Here's the drawing with two shaded views (mm, measured from the low corner). I have some questions. Give positions to 0.01 mm unless a question says otherwise; leave off trailing zeros. Loops run counter-clockwise (first coordinate to the right, second up) from the corner with the lowest first, then second, coordinate; pieces in that order, holes last.
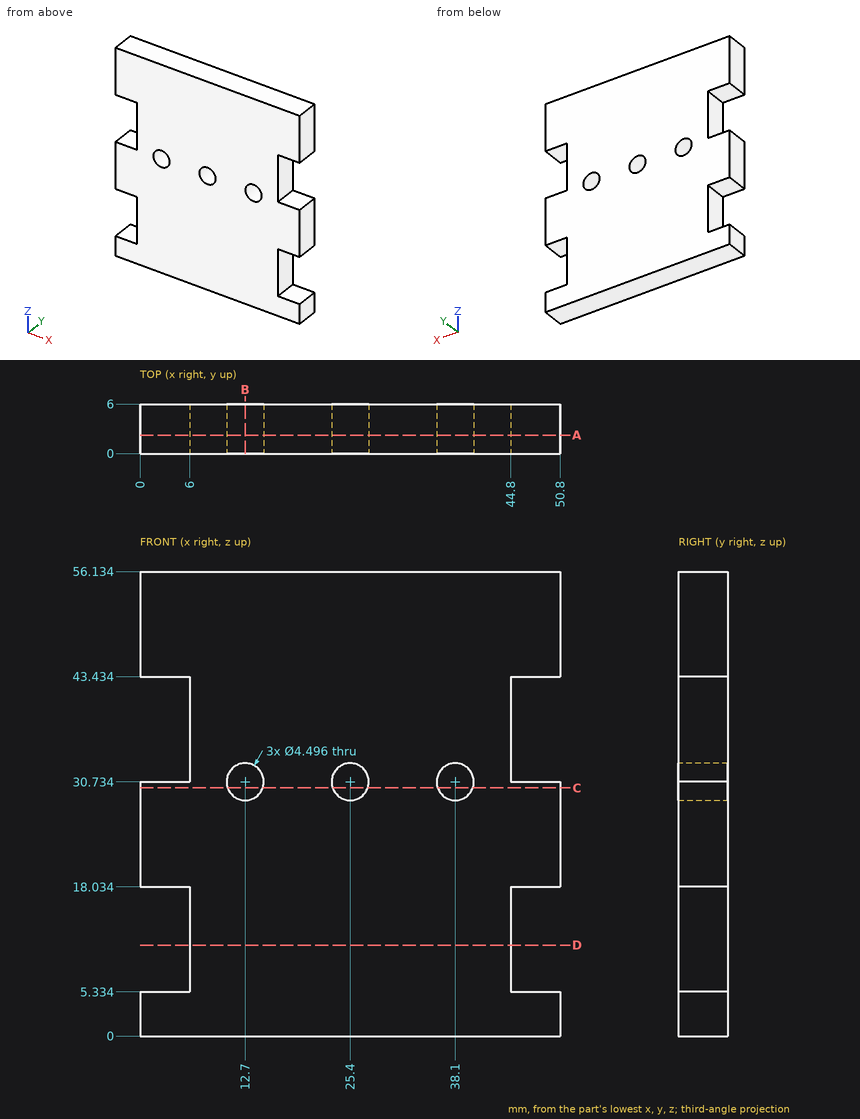
(1) Please list where these lines run through material, in increasing order: probe 1 along X at (y, z) = (2.5, 29); probe 2 along Z at (x, y) = (38.1, 2.35); probe 3 along X at (y, z) = (2, 12).
Returned:
probe 1: x = 0 to 11.27, 14.13 to 23.97, 26.83 to 36.67, 39.53 to 50.8
probe 2: z = 0 to 28.49, 32.98 to 56.13
probe 3: x = 6 to 44.8
(2) Will these pins go through, and if not, where does the flat tip stop? P1, Ø1.8, axis at y = 4, z = 36.5, coming from the +X side; P2, Ø1.8, axis at y = 2.5, z = 10.5, coming from the -X side.
Returned:
P1: stops at x = 44.8
P2: stops at x = 6
(3) Suppose I cut it at D-D on z = 11. List the corners of the cut face in (x, y) for me.
Returned:
outline: (6, 0) - (44.8, 0) - (44.8, 6) - (6, 6) - close
(4) Suppose I cut it at C-C on z = 30. List the corners of the cut face in (x, y) for me (1 decimal), plus the area to 3 significant figures.
Returned:
outline: (0, 0) - (10.6, 0) - (10.6, 6) - (0, 6) - close; (14.8, 0) - (23.3, 0) - (23.3, 6) - (14.8, 6) - close; (27.5, 0) - (36, 0) - (36, 6) - (27.5, 6) - close; (40.2, 0) - (50.8, 0) - (50.8, 6) - (40.2, 6) - close
area: 228 mm2
(5) Suppose I cut it at A-A on y = 2.25. List the corners of the cut face in (x, z) for me.
Returned:
outline: (0, 0) - (50.8, 0) - (50.8, 5.33) - (44.8, 5.33) - (44.8, 18.03) - (50.8, 18.03) - (50.8, 30.73) - (44.8, 30.73) - (44.8, 43.43) - (50.8, 43.43) - (50.8, 56.13) - (0, 56.13) - (0, 43.43) - (6, 43.43) - (6, 30.73) - (0, 30.73) - (0, 18.03) - (6, 18.03) - (6, 5.33) - (0, 5.33) - close; hole circle Ø4.5 at (12.7, 30.73); hole circle Ø4.5 at (25.4, 30.73); hole circle Ø4.5 at (38.1, 30.73)
(6) Suppose I cut it at B-B on x = 12.7. List the corners of the cut face in (y, z) for me.
Returned:
outline: (0, 0) - (6, 0) - (6, 28.49) - (0, 28.49) - close; (0, 32.98) - (6, 32.98) - (6, 56.13) - (0, 56.13) - close
